from build123d import *

# Parameters (mm, degrees)
F1_DEPTH = 15.875
F2_R     = 4.572
F3_SIZE  = 5.08


with BuildPart() as f1:
    # F0 (on Front) → F1 (new body, symmetric)
    with BuildSketch(Plane.XZ):
        Polygon((0, 41.275), (0, 0), (6.35, 0), (6.35, 34.925), (38.1, 34.925), (38.1, 41.275), align=None)
    extrude(amount=F1_DEPTH, both=True)

    # F2
    f2_edges = [f1.edges().sort_by_distance(p)[0] for p in [
        (6.35, 0, 34.925),
    ]]
    fillet(f2_edges, radius=F2_R)

    # F3
    f3_edges = [f1.edges().sort_by_distance(p)[0] for p in [
        (3.175, 15.875, 0),
    ]]
    chamfer(f3_edges, length=F3_SIZE)


solid = f1.part
Design review of the part built by this model. Coordinates are the model's own, in mm. A direction names the side the tool comes from. Round coordinates to 2 decimals unless told otherwise and drop trailing zeros. Write each loop counter-clockwise with the first axis right and the second up, starting at its lowest first coordinate (ties: lowest second). Pieces come first, ordered by that corner, then holes. Notation, with made-up numbers: (26.5, 28.5) -> (31.5, 28.5) arc R11 cw to (31.5, 47.5) -> close; hole circle Ø5 at (87.5, 10.5). An arc over 180 degrees is marked (long way). One line per question, with ' | ' between items.
(1) Insertion check: P1, Ø6, axis at x = 27.5, y = 8, coming from the -Z side (3 decimals); P2, Ø8, axis at x = 11, y = 0.5, coming from the -Z side; P3, Ø15, axis at y = 6, z = 14.5, coming from the +X side. Each pin has a flat end and moves straight along its axis. Give the tip position at first contact, or say it passes through.
Result sheet:
P1: z = 34.925 | P2: z = 32.7 | P3: x = 6.35
(2) Take a section at C-C, the plane z = 15.5. State the section outline as (x, y) points (3 decimals), and give its area (3 significant figures).
Result sheet:
outline: (0, -15.875) -> (6.35, -15.875) -> (6.35, 15.875) -> (0, 15.875) -> close | area: 202 mm2
(3) Wall thickness on line 1 (X direction, y = 3.5, z = 18.5); line 2 (Z direction, x = 27.5, y = -5) (3 decimals): over which ranges is each line inside the solid? List them lowest first. Write a range as [from, to].
Result sheet:
line 1: [0, 6.35] | line 2: [34.925, 41.275]
(4) Take a section at A-A, the plane y = 8. State the section outline as (x, z) points (3 decimals), and give its area (3 significant figures).
Result sheet:
outline: (0, 0) -> (6.35, 0) -> (6.35, 30.353) arc R4.572 cw to (10.922, 34.925) -> (38.1, 34.925) -> (38.1, 41.275) -> (0, 41.275) -> close | area: 468 mm2
(5) Take a section at D-D, the plane y = 14. State the section outline as (x, z) points (3 decimals).
Result sheet:
outline: (0, 3.205) -> (6.35, 3.205) -> (6.35, 30.353) arc R4.572 cw to (10.922, 34.925) -> (38.1, 34.925) -> (38.1, 41.275) -> (0, 41.275) -> close
(6) Draft analysis for pull direction Y (two halves, no side actions). For faces 3 (the flat face through (10, 15.875, 35)), 4 (the flat face through (6, -15.875, 27)), 5 (the flat face through (3, -3, 0)), state which applies: released by +Y, released by -Y, zero draft, split by the parting line, or undercut.
Result sheet:
face 3: released by +Y | face 4: released by -Y | face 5: zero draft
(7) Machinability: for faces 1 (the flat face through (6.35, 0, 15)), 2 (the flat face through (3.131, 13.299, 2.504)), which of the approach directions +Z, -Z, +X, -X, +Y, -Y give a long, thin tool a straight path to every point of the face, cutting with its end or side? Answer none if there is none.
Result sheet:
face 1: -Z, +X, +Y, -Y | face 2: -Z, +X, -X, +Y
(8) Take a section at B-B, the plane x = 12.5. State the section outline as (y, z) points (3 decimals), and give its area (3 significant figures).
Result sheet:
outline: (-15.875, 34.925) -> (15.875, 34.925) -> (15.875, 41.275) -> (-15.875, 41.275) -> close | area: 202 mm2
